The listing builds one solid part. Answer for the finished solid, in the listing's coordinates (mm). Round coordinates to 2 decimals unless told otherwise and drop trailing zeros. Write each loop counter-clockwise with the first axis right and the second up, starting at its lowest first coordinate (ties: lowest second). Pieces come first, ordered by that corner, then holes.
from build123d import *


with BuildPart() as part:
    # Washer Revolve Profile → Washer Revolve (revolve)
    with BuildSketch(Plane.XY, mode=Mode.PRIVATE) as washer_revolve_sk:
        Polygon((2.159, 2.667), (2.159, 0), (3.175, 0), (3.175, 1.397), (4.7625, 1.397), (4.7625, 2.413), (4.5085, 2.667), align=None)
    revolve(washer_revolve_sk.sketch.rotate(Axis((0, 0, 0), (0, 1, 0)), 90), axis=Axis((0, 0, 0), (0, 1, 0)))


solid = part.part
1. For a pull along X with two mould halves and no side action, classify faces 1 (the face through (1.93, 0.71, 2.52)), 2 (the face through (-2.1, 2.667, 1.1)), 3 (the face through (-2.14, 1.31, 0.28)) as released by +X, released by -X, zero draft, split by the parting line, or undercut.
Geometry says:
face 1: split by the parting line
face 2: zero draft
face 3: undercut
2. Section D-D on y = 1.95 is taken. Determine the outline of the cut face in (x, z) (1 decimal).
Geometry says:
outline: circle Ø9.5 at (0, 0); hole circle Ø4.3 at (0, 0)
3. Section C-C on y = 1.05 is taken. Determine the outline of the cut face in (x, z) (3 decimals).
Geometry says:
outline: circle Ø6.35 at (0, 0); hole circle Ø4.318 at (0, 0)
4. Straight lines are drawn through the part: line 1 along X through (y, z) = (1.7, 0); line 2 along X through (y, z) = (1.2, 0) (3 decimals); line 3 along Y through (x, z) = (-0.25, 4). For each, find the intervals that lie inside material, in ascending order.
Geometry says:
line 1: x = -4.76 to -2.16, 2.16 to 4.76
line 2: x = -3.175 to -2.159, 2.159 to 3.175
line 3: y = 1.4 to 2.67
